The listing builds one solid part. Answer for the finished solid, in the listing's coordinates (mm). Coordinates: 2 decimals unless noted, no trailing zeros. Write each loop counter-clockwise with the first axis right and the second up, starting at its lowest first coordinate (ties: lowest second). Pieces come first, ordered by that corner, then holes.
(1) The part is cut by section A-A on z = 0. Determine the outline of the cut face in (x, y), plus the area to 3 significant figures.
(2) The part is cut by section C-C on x = 185.5. Determine the outline of the cut face in (y, z), plus the area to 3 significant figures.
(3) The part is cut by section D-D on z = 278. Determine the outline of the cut face in (x, y).
(4) Given P1, Ø17.5, axis at x = -225.08, z = 389.86, coming from the +Y side; P2, Ø8, axis at x = -298, z = -3.5, coming from the -Y side; P3, Ø5, axis at y = 1.5, z = -117.5, coming from the +X side; P4, Ø1, axis at y = 8.5, z = 272.5, coming from the -X side, each flat-ended and moving along its own axis, determine where each tip first touches the part or whether it passes through.
(5) Straight lines are drawn through the part: line 1 (X direction, y = 3.75, z = -1.5); line 2 (X direction, y = 5.75, z = -335); line 3 (Z direction, x = -350, y = 11.5). For each, find the intervals that lie inside material, in ascending order.
(6) The part is cut by section B-B on x = 0. Determine the outline of the cut face in (y, z).
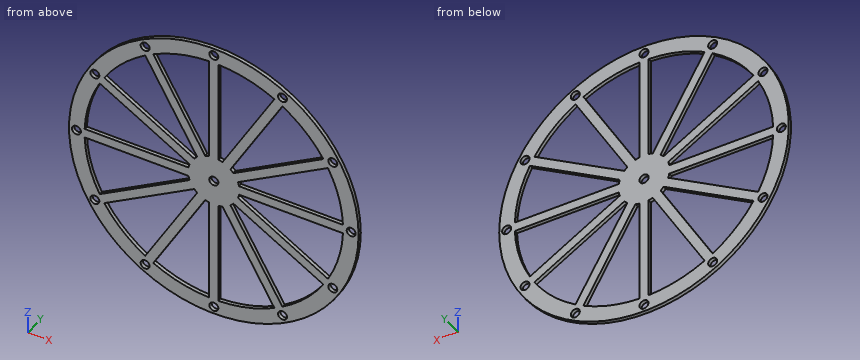
from build123d import *

# Parameters (mm, degrees)
SKETCH1_R            = 474.432327188
SKETCH1_R_2          = 15
SKETCH1_R_3          = 14.738282491
BOSS_EXTRUDE15_DEPTH = 12


with BuildPart() as part:
    # Sketch1 → Boss-Extrude15 (new body)
    with BuildSketch(Plane(origin=(0, 0, 0), x_dir=(1, 0, 0), z_dir=(0, 1, 0))):
        Circle(SKETCH1_R)
        Circle(SKETCH1_R_2, mode=Mode.SUBTRACT)
        with Locations((0, 450.168808025)):
            Circle(SKETCH1_R_3, mode=Mode.SUBTRACT)
        with Locations((225.084404013, 389.857623741)):
            Circle(SKETCH1_R_3, mode=Mode.SUBTRACT)
        with Locations((389.857623741, 225.084404013)):
            Circle(SKETCH1_R_3, mode=Mode.SUBTRACT)
        with Locations((450.168808025, 0)):
            Circle(SKETCH1_R_3, mode=Mode.SUBTRACT)
        with Locations((389.857623741, -225.084404013)):
            Circle(SKETCH1_R_3, mode=Mode.SUBTRACT)
        with Locations((225.084404013, -389.857623741)):
            Circle(SKETCH1_R_3, mode=Mode.SUBTRACT)
        with Locations((0, -450.168808025)):
            Circle(SKETCH1_R_3, mode=Mode.SUBTRACT)
        with Locations((-225.084404012, -389.857623741)):
            Circle(SKETCH1_R_3, mode=Mode.SUBTRACT)
        with Locations((-389.857623741, -225.084404013)):
            Circle(SKETCH1_R_3, mode=Mode.SUBTRACT)
        with Locations((-450.168808025, 0)):
            Circle(SKETCH1_R_3, mode=Mode.SUBTRACT)
        with Locations((-389.857623741, 225.084404013)):
            Circle(SKETCH1_R_3, mode=Mode.SUBTRACT)
        with Locations((-225.084404013, 389.857623741)):
            Circle(SKETCH1_R_3, mode=Mode.SUBTRACT)
        with BuildLine():
            Line((15.084021598, 423.182152072), (15.084021598, 82.782783758))
            ThreePointArc((15.084021598, 82.782783758), (21.778537661, 81.278609065), (28.328245984, 79.234004529))
            Line((28.328245984, 79.234004529), (198.527930141, 374.028504921))
            ThreePointArc((198.527930141, 374.028504921), (109.597156617, 409.022156859), (15.084021598, 423.182152072))
        make_face(mode=Mode.SUBTRACT)
        with BuildLine():
            Line((-15.084021598, 423.182152072), (-15.084021598, 82.782783758))
            ThreePointArc((-15.084021598, 82.782783758), (-21.778537661, 81.278609065), (-28.328245984, 79.234004529))
            Line((-28.328245984, 79.234004529), (-198.527930141, 374.028504921))
            ThreePointArc((-198.527930141, 374.028504921), (-109.597156617, 409.022156859), (-15.084021598, 423.182152072))
        make_face(mode=Mode.SUBTRACT)
        with BuildLine():
            Line((224.654221931, 358.944483323), (54.454537774, 64.149982931))
            ThreePointArc((54.454537774, 64.149982931), (59.500071404, 59.500071404), (64.149982931, 54.454537774))
            Line((64.149982931, 54.454537774), (358.944483323, 224.654221931))
            ThreePointArc((358.944483323, 224.654221931), (299.425000242, 299.425000242), (224.654221931, 358.944483323))
        make_face(mode=Mode.SUBTRACT)
        with BuildLine():
            Line((374.028504921, 198.527930141), (79.234004529, 28.328245984))
            ThreePointArc((79.234004529, 28.328245984), (81.278609065, 21.778537661), (82.782783758, 15.084021598))
            Line((82.782783758, 15.084021598), (423.182152072, 15.084021598))
            ThreePointArc((423.182152072, 15.084021598), (409.022156859, 109.597156617), (374.028504921, 198.527930141))
        make_face(mode=Mode.SUBTRACT)
        with BuildLine():
            Line((423.182152072, -15.084021598), (82.782783758, -15.084021598))
            ThreePointArc((82.782783758, -15.084021598), (81.278609065, -21.778537661), (79.234004529, -28.328245984))
            Line((79.234004529, -28.328245984), (374.028504921, -198.527930141))
            ThreePointArc((374.028504921, -198.527930141), (409.022156859, -109.597156617), (423.182152072, -15.084021598))
        make_face(mode=Mode.SUBTRACT)
        with BuildLine():
            Line((358.944483323, -224.654221931), (64.149982931, -54.454537774))
            ThreePointArc((64.149982931, -54.454537774), (59.500071404, -59.500071404), (54.454537774, -64.149982931))
            Line((54.454537774, -64.149982931), (224.654221931, -358.944483323))
            ThreePointArc((224.654221931, -358.944483323), (299.425000242, -299.425000242), (358.944483323, -224.654221931))
        make_face(mode=Mode.SUBTRACT)
        with BuildLine():
            Line((198.527930141, -374.028504921), (28.328245984, -79.234004529))
            ThreePointArc((28.328245984, -79.234004529), (21.778537661, -81.278609065), (15.084021598, -82.782783758))
            Line((15.084021598, -82.782783758), (15.084021598, -423.182152072))
            ThreePointArc((15.084021598, -423.182152072), (109.597156617, -409.022156859), (198.527930141, -374.028504921))
        make_face(mode=Mode.SUBTRACT)
        with BuildLine():
            Line((-15.084021598, -423.182152072), (-15.084021598, -82.782783758))
            ThreePointArc((-15.084021598, -82.782783758), (-21.778537661, -81.278609065), (-28.328245984, -79.234004529))
            Line((-28.328245984, -79.234004529), (-198.527930141, -374.028504921))
            ThreePointArc((-198.527930141, -374.028504921), (-109.597156617, -409.022156859), (-15.084021598, -423.182152072))
        make_face(mode=Mode.SUBTRACT)
        with BuildLine():
            Line((-224.654221931, -358.944483323), (-54.454537774, -64.149982931))
            ThreePointArc((-54.454537774, -64.149982931), (-59.500071404, -59.500071404), (-64.149982931, -54.454537774))
            Line((-64.149982931, -54.454537774), (-358.944483323, -224.654221931))
            ThreePointArc((-358.944483323, -224.654221931), (-299.425000242, -299.425000242), (-224.654221931, -358.944483323))
        make_face(mode=Mode.SUBTRACT)
        with BuildLine():
            Line((-374.028504921, -198.527930141), (-79.234004529, -28.328245984))
            ThreePointArc((-79.234004529, -28.328245984), (-81.278609065, -21.778537661), (-82.782783758, -15.084021598))
            Line((-82.782783758, -15.084021598), (-423.182152072, -15.084021598))
            ThreePointArc((-423.182152072, -15.084021598), (-409.022156859, -109.597156617), (-374.028504921, -198.527930141))
        make_face(mode=Mode.SUBTRACT)
        with BuildLine():
            Line((-423.182152072, 15.084021598), (-82.782783758, 15.084021598))
            ThreePointArc((-82.782783758, 15.084021598), (-81.278609065, 21.778537661), (-79.234004529, 28.328245984))
            Line((-79.234004529, 28.328245984), (-374.028504921, 198.527930141))
            ThreePointArc((-374.028504921, 198.527930141), (-409.022156859, 109.597156617), (-423.182152072, 15.084021598))
        make_face(mode=Mode.SUBTRACT)
        with BuildLine():
            Line((-358.944483323, 224.654221931), (-64.149982931, 54.454537774))
            ThreePointArc((-64.149982931, 54.454537774), (-59.500071404, 59.500071404), (-54.454537774, 64.149982931))
            Line((-54.454537774, 64.149982931), (-224.654221931, 358.944483323))
            ThreePointArc((-224.654221931, 358.944483323), (-299.425000242, 299.425000242), (-358.944483323, 224.654221931))
        make_face(mode=Mode.SUBTRACT)
    extrude(amount=BOSS_EXTRUDE15_DEPTH)


solid = part.part
Model answer:
1. outline: (-474.43, 0) - (-464.91, 0) - (-464.91, 12) - (-474.43, 12) - close; (-435.43, 0) - (-15, 0) - (-15, 12) - (-435.43, 12) - close; (15, 0) - (435.43, 0) - (435.43, 12) - (15, 12) - close; (464.91, 0) - (474.43, 0) - (474.43, 12) - (464.91, 12) - close
1. area: 10,300 mm2
2. outline: (0, -436.66) - (12, -436.66) - (12, -380.66) - (0, -380.66) - close; (0, -351.46) - (12, -351.46) - (12, -291.13) - (0, -291.13) - close; (0, -124.52) - (12, -124.52) - (12, -89.68) - (0, -89.68) - close; (0, -15.08) - (12, -15.08) - (12, 15.08) - (0, 15.08) - close; (0, 89.68) - (12, 89.68) - (12, 124.52) - (0, 124.52) - close; (0, 291.13) - (12, 291.13) - (12, 351.46) - (0, 351.46) - close; (0, 380.66) - (12, 380.66) - (12, 436.66) - (0, 436.66) - close
2. area: 3,990 mm2
3. outline: (-384.45, 0) - (-319.42, 0) - (-319.42, 12) - (-384.45, 12) - close; (-177.92, 0) - (-143.09, 0) - (-143.09, 12) - (-177.92, 12) - close; (-15.08, 0) - (15.08, 0) - (15.08, 12) - (-15.08, 12) - close; (143.09, 0) - (177.92, 0) - (177.92, 12) - (143.09, 12) - close; (319.42, 0) - (384.45, 0) - (384.45, 12) - (319.42, 12) - close
4. P1: passes through
4. P2: stops at y = 0
4. P3: stops at x = 460.28
4. P4: stops at x = -388.72
5. line 1: x = -474.43 to -464.83, -435.51 to -14.92, 14.92 to 435.51, 464.83 to 474.43
5. line 2: x = -335.95 to -259.01, -210.83 to -175.99, -15.08 to 15.08, 175.99 to 210.83, 259.01 to 335.95
5. line 3: z = -320.29 to -238.35, -219.49 to -184.66, -15.08 to 15.08, 184.66 to 219.49, 238.35 to 320.29
6. outline: (0, -474.43) - (12, -474.43) - (12, -464.91) - (0, -464.91) - close; (0, -435.43) - (12, -435.43) - (12, -15) - (0, -15) - close; (0, 15) - (12, 15) - (12, 435.43) - (0, 435.43) - close; (0, 464.91) - (12, 464.91) - (12, 474.43) - (0, 474.43) - close
